from build123d import *

# Parameters (mm, degrees)
ESQUISSE1_W        = 100
ESQUISSE1_H        = 1.65
EXTRU_MINCE1_DEPTH = 60
EXTRU_MINCE2_DEPTH = 60
CONG_1_SIZE        = 15
CONG_1_SIZE_2      = 60


# Read off the part's stored shape, not the designer's step: Extru.-Mince2
with BuildPart() as part:
    # Esquisse1 → Extru.-Mince1 (new body)
    with BuildSketch(Plane.XY):
        with Locations((50, 0.825)):
            Rectangle(ESQUISSE1_W, ESQUISSE1_H)
    extrude(amount=EXTRU_MINCE1_DEPTH)

    # Extru.-Mince2 outline → Extru.-Mince2 (add)
    with BuildSketch(Plane.XY):
        Polygon((-30, 0), (0, 0), (0, 1.65), (3.2, 1.65), (3.2, 200), (0, 200), (0, 3.2), (-30, 3.2), align=None)
    extrude(amount=EXTRU_MINCE2_DEPTH)

    # Congé1
    # an asymmetric fillet: 60, 15 mm, written as the material it adds along each edge
    with BuildSketch(Plane(origin=(0, 3.2, 0), x_dir=(-1, 0, 0), z_dir=(0, 0, 1))) as cong_1_piece_1:
        with BuildLine():
            Bezier((CONG_1_SIZE, 0), (0, 0), (0, -CONG_1_SIZE_2), weights=[1, 0.707106781, 1])
            Line((0, -CONG_1_SIZE_2), (0, 0))
            Line((0, 0), (CONG_1_SIZE, 0))
        make_face()
    extrude(amount=60)


solid = part.part
Input: part model. Units: mm. Frame: model coordinates. A direction names the side the tool comes from. Round coordinates to 2 decimals unless told otherwise and drop trailing zeros. Order: outer loops, then holes, each group sorted by start corner. A loop starts at its lowest first (then second) coordinate and runs counter-clockwise, first axis right, second up. Notation, with made-up numbers: (-18.75, 32.5) - (-12.75, 32.5) arc R29 cw to (-12.75, 67.5) - close; hole circle Ø8 at (33.25, 3.25). An arc over 180 degrees is marked (long way). Answer as a JSON object with one key per item and string values. Group by question number.
(1) Cut plane A-A (x = 77). Return loops of the section in (y, z).
(2) Cut plane B-B (y = 115.5). Return loops of the section in (x, z), then the cut area to 3 significant figures.
(3) Pin query (flat end, axial travel): P1, Ø12, axis at y = 128, z = 17, coming from the +X side; P2, Ø4, axis at x = 67, z = 22.5, coming from the +Y side; P3, Ø6, axis at y = 42.5, z = 52, coming from the -X side. Return the tip coordinate at first contact, or that it passes through.
(4) Reachability of faces 1 (the face through (51, 1.65, 30)), 2 (the face through (1, 85, 60)), 3 (the face through (0, 133, 30)) from +Z, -Z, +X, -X, +Y, -Y: full face, straight path, thin tool, end or side. Return the list, or none.
(5) Material intervals for probe 1 along Y at (x, z) = (33.5, 28); probe 2 along Y at (x, z) = (-14.5, 31); probe 3 along X at (y, z) = (83.5, 5.5), sorted ascending. Write a range as from..to.
Here are the results:
{
 "1": {"outline": "(0, 0) - (1.65, 0) - (1.65, 60) - (0, 60) - close"},
 "2": {"outline": "(0, 0) - (3.2, 0) - (3.2, 60) - (0, 60) - close", "area": "192 mm^2"},
 "3": {"P1": "stops at x = 3.2", "P2": "stops at y = 1.65", "P3": "stops at x = -1.22"},
 "4": {"face 1": "+Z, -Z, +X, +Y", "face 2": "+Z, +X, -X, +Y, -Y", "face 3": "+Z, -Z, -X, +Y"},
 "5": {"probe 1": "y = 0..1.65", "probe 2": "y = 0..3.23", "probe 3": "x = 0..3.2"}
}
